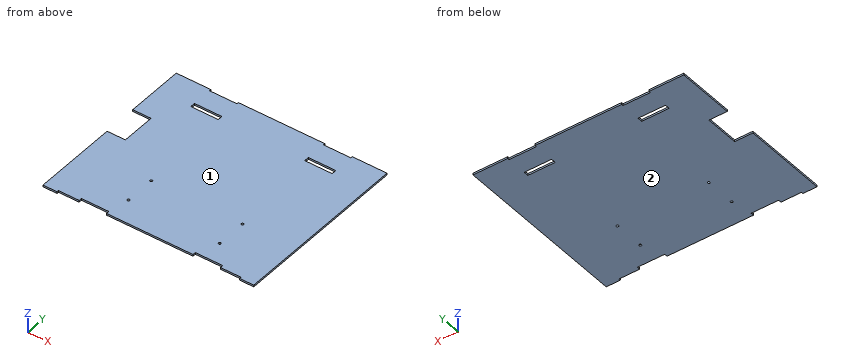
```python
from build123d import *

# Parameters (mm, degrees)
SCHIZZO1_W                    = 45
SCHIZZO1_H                    = 8
ESTRUSIONE_ESTRUSIONE1_DEPTH  = 3
TAGLIO_ESTRUSIONE1_DEPTH      = 228.039644115
TAGLIO_ESTRUSIONE1_DEPTH_BACK = 228.039644115
SCHIZZO2_R                    = 2
SCHIZZO3_W                    = 30
SCHIZZO3_H                    = 56
TAGLIO_ESTRUSIONE2_DEPTH      = 228.039644115


with BuildPart() as part:
    # Schizzo1 → Estrusione-Estrusione1 (new body)
    with BuildSketch(Plane.XY):
        Polygon((173, -147), (173, 144), (116, 144), (116, 141), (71, 141), (71, 144), (-71, 144), (-71, 141), (-116, 141), (-116, 144), (-173, 144), (-173, -147), (-150, -147), (-150, -144), (-116, -144), (-116, -139), (-71, -139), (-71, -144), (71, -144), (71, -139), (116, -139), (116, -144), (150, -144), (150, -147), align=None)
        with Locations((93.5, 104)):
            Rectangle(SCHIZZO1_W, SCHIZZO1_H, mode=Mode.SUBTRACT)
        with Locations((-93.5, 104)):
            Rectangle(SCHIZZO1_W, SCHIZZO1_H, mode=Mode.SUBTRACT)
    extrude(amount=ESTRUSIONE_ESTRUSIONE1_DEPTH)

    # Schizzo2 → Taglio-Estrusione1 (cut, two sides: drawn at the far end of the back side and taken through both)
    with BuildSketch(Plane.XY.offset(3).offset(-TAGLIO_ESTRUSIONE1_DEPTH_BACK)):
        with Locations((-64.85, -54.5)):
            Circle(SCHIZZO2_R)
        with Locations((85.15, -54.5)):
            Circle(SCHIZZO2_R)
        with Locations((85.15, -104.5)):
            Circle(SCHIZZO2_R)
        with Locations((-64.85, -104.5)):
            Circle(SCHIZZO2_R)
    extrude(amount=TAGLIO_ESTRUSIONE1_DEPTH + TAGLIO_ESTRUSIONE1_DEPTH_BACK, mode=Mode.SUBTRACT)

    # Schizzo3 → Taglio-Estrusione2 (cut, through all)
    with BuildSketch(Plane(origin=(0, 0, 0), x_dir=(-1, 0, 0), z_dir=(0, 0, -1))):
        with Locations((158, 21)):
            Rectangle(SCHIZZO3_W, SCHIZZO3_H)
    extrude(amount=-TAGLIO_ESTRUSIONE2_DEPTH, mode=Mode.SUBTRACT)


solid = part.part
```
Geometry check sheet. Reference: the model listing, model coordinates, mm. Face numbers are marked on the shaded views. Coordinates: 2 decimals unless noted, no trailing zeros. Order: outer loops, then holes, each group sorted by start corner. A loop starts at its lowest first (then second) coordinate and runs counter-clockwise, first axis right, second up. Notation, with made-up numbers: M 57,-35 L 83,-35 A10 cw 83,-18 Z; hole C 88,-25 d2. An arc over 180 degrees is marked long. One line per question, with ' | ' between items. Start each with the question number.
Item 1: Draft check along Z on the marked faces 1 and 2. Enter one of: pulls with the +Z half, pulls with the -Z half, needs draft (parallel to the pull), parting line crosses it, or undercut.
Item 2: Cross-section at C-C on y = 0. Enter the section's corners in (x, z).
Item 3: Cross-section at B-B on z = 1.45. State how many separate pieces and enclosed holes the cut face has, then the cut area to 3 significant figures.
Item 4: Cross-section at A-A on x = -112. Enter the section's corners in (y, z), then the cut area to 3 significant figures.
Item 5: Material ranges on L1, parallel to X at y = -104.5, z = 1.35; L2, parallel to Y at x = -64.85, z = 1.5; L3, parallel to Y at x = 104, z = 2.05, recorded low to high. Write a range as [from, to].
Item 6: Gauge pin test, flat ends, axial feed: pin 1 (3.5 mm diameter, centred on x = -64.85, y = -54.5, fed in from +Z); pin 2 (0.9 mm diameter, centred on x = -98, z = 1.5, fed in from +Y). Record the tip position at first contact, or that the pin passes through.
Findings:
1) face 1: pulls with the +Z half | face 2: pulls with the -Z half
2) outline: M -143,0 L 173,0 L 173,3 L -143,3 Z
3) separate pieces: 1 | enclosed holes: 6 | area: 96,600 mm²
4) outline: M -139,0 L 100,0 L 100,3 L -139,3 Z; M 108,0 L 141,0 L 141,3 L 108,3 Z | area: 816 mm²
5) L1: x = [-173, -66.85], [-62.85, 83.15], [87.15, 173] | L2: y = [-144, -106.5], [-102.5, -56.5], [-52.5, 144] | L3: y = [-139, 100], [108, 141]
6) pin 1: passes through | pin 2: stops at y = 141
